Study the drawing (mm; zero at the part's minimum x, y, z) and answer. A direction names the side the tool comes from. Give positions to 0.01 mm unless a question says otherwise; leave off trailing zeros. Loops run counter-clockwise (first coordinate to the right, second up) from the corner with the lowest first, then second, coordinate; pieces in that order, holes last. Notation, with made-up numbers: (-32.75, 52.25) - (8.25, 52.25) arc R34 cw to (8.25, 91.25) - close; hole circle Ø8 at (-34, -37.5). An arc over 180 degrees is marked (long way). Write item = value, one per line. Start each with the question number.
1) Which of the six approach directions +Z, -Z, +X, -X, +Y, -Y give full straight-line access (tool end or side, diameter ignored) to the marked faces 5, 6 and 7?
2) The part is cut by section D-D on y = 3. Write down the section's boundary in (x, z), plus the area to 3 significant figures.
3) Consider probe 1 along Y at (x, z) = (9.25, 4.25); probe 2 along X at (y, z) = (2, 3.25); probe 3 along X at (y, z) = (11.75, 9). Determine where each line is inside the solid, lowest interval first.
4) Flat-ended cylindrical pins translate along their axes: P1, Ø1.3, axis at y = 1.5, z = 10.5, coming from the +X side; P2, Ø3.5, axis at x = 17, z = 6.5, coming from the +Y side; P3, Ø2.5, axis at x = 17.5, z = 11.5, coming from the -Y side. Find the tip coordinate at first contact, or state that the pin passes through.
5) The part is cut by section A-A on x = 3.75. Write down the section's boundary in (y, z).
6) The part is cut by section B-B on z = 25.5. Write down the section's boundary in (x, y).
7) The mould has two halves that part along Y. Classify the marked faces 1, 2, 3 and 4: +Y half, -Y half, draft (parallel to the pull), parting line (faces both ways), or undercut.
8) The part is cut by section C-C on z = 7. Write down the section's boundary in (x, y), plus the area to 3 significant figures.
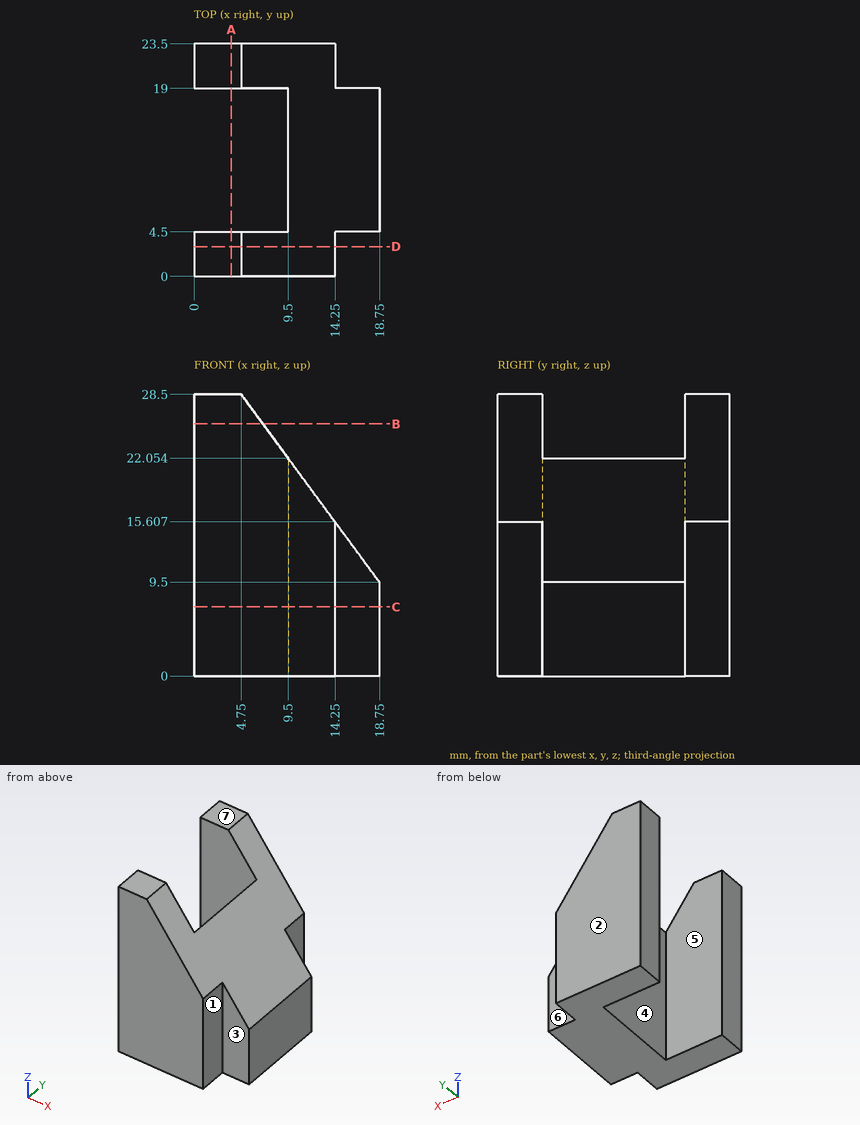
Answer below:
q1.face_5 = +Z, -Z, -X
q1.face_6 = +Z, -Z, +X, +Y
q1.face_7 = +Z, +X, -X, +Y, -Y
q2.outline = (0, 0) - (14.25, 0) - (14.25, 15.61) - (4.75, 28.5) - (0, 28.5) - close
q2.area = 345 mm2
q3.probe_1 = 0 to 4.5, 19 to 23.5
q3.probe_2 = 0 to 14.25
q3.probe_3 = 9.5 to 18.75
q4.P1 = 14.25
q4.P2 = 19
q4.P3 = 4.5
q5.outline = (0, 0) - (4.5, 0) - (4.5, 28.5) - (0, 28.5) - close; (19, 0) - (23.5, 0) - (23.5, 28.5) - (19, 28.5) - close
q6.outline = (0, 0) - (6.96, 0) - (6.96, 4.5) - (0, 4.5) - close; (0, 19) - (6.96, 19) - (6.96, 23.5) - (0, 23.5) - close
q7.face_1 = draft
q7.face_2 = +Y half
q7.face_3 = -Y half
q7.face_4 = undercut
q8.outline = (0, 0) - (14.25, 0) - (14.25, 4.5) - (18.75, 4.5) - (18.75, 19) - (14.25, 19) - (14.25, 23.5) - (0, 23.5) - (0, 19) - (9.5, 19) - (9.5, 4.5) - (0, 4.5) - close
q8.area = 262 mm2
